Here's how the part is built. I have some questions about the finished solid (model axes, mm). Face numbers are marked on the shaded views. A direction names the side the tool comes from. Coordinates: 2 decimals unless noted, no trailing zeros. Write each loop counter-clockwise with the first axis right and the second up, starting at its lowest first coordinate (ties: lowest second). Pieces come first, ordered by that corner, then holes.
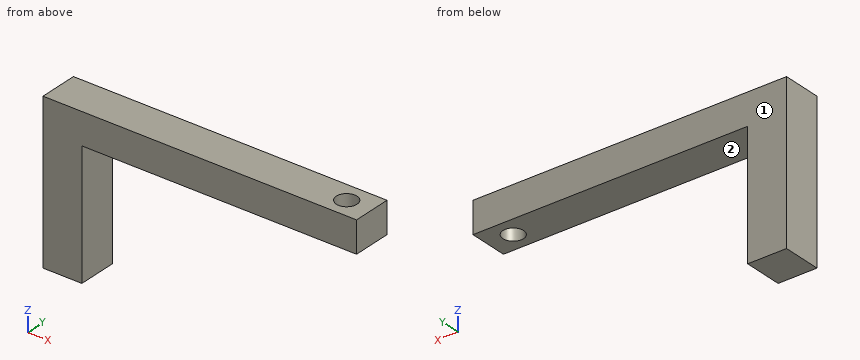
from build123d import *

# Parameters (mm, degrees)
F0_W     = 6.2
F0_H     = 6.2
F1_DEPTH = 20
F2_W     = 50
F2_H     = 6.2
F3_DEPTH = 5
F4_R     = 1.65
F5_DEPTH = 25


with BuildPart() as f1:
    # F0 (on Top) → F1 (new body)
    with BuildSketch(Plane.XY):
        Rectangle(F0_W, F0_H)
    extrude(amount=F1_DEPTH)

    # F2 (on face) → F3 (join)
    with BuildSketch(Plane.XY.offset(20)):
        with Locations((21.9, 0)):
            Rectangle(F2_W, F2_H)
    extrude(amount=F3_DEPTH)

    # F4 (on face) → F5 (cut)
    with BuildSketch(Plane.XY.offset(25)):
        with Locations((42.9, 0)):
            Circle(F4_R)
    extrude(amount=-F5_DEPTH, mode=Mode.SUBTRACT)


solid = f1.part
1. I want a section at B-B (x = 42.9). List the corners of the cut face in (y, z) for me.
2. On a 3-axis mill with a long thin cutter (end or side, diameter ignored), from which of +Z, -Z, +X, -X, +Y, -Y can I reach the whole of each face in a straight line? I mean the marked faces 1 and 2. Say none if no direction works.
3. If I drill on line 1 (Y direction, x = 42.9, z = 22.75); line 2 (X direction, y = -2.75, z = 8.5); line 3 (Z direction, x = 23, y = -0.75), over which ranges is the centre line in solid material (lowest first)?
4. I want a section at A-A (y = 0). List the corners of the cut face in (x, z) for me, then the cut area to 4 significant figures.
5. I want a section at D-D (y = -2.5). List the corners of the cut face in (x, z) for me.
6. I want a section at C-C (z = 20.75). List the corners of the cut face in (x, y) for me, then the cut area to 3 significant figures.
7. For pin 1 Ø1.9 at (y, z) = (0.5, 14.5) entering from +X; pin 2 Ø3 at (x, y) = (23, 1) entering from -Z, each with a flat end and sliding along its axis, tell me the tip position at first contact or that it passes through.
Response values:
1. outline: (-3.1, 20) - (-1.65, 20) - (-1.65, 25) - (-3.1, 25) - close; (1.65, 20) - (3.1, 20) - (3.1, 25) - (1.65, 25) - close
2. face 1: +Z, -Z, +X, -X, +Y
2. face 2: -Z, +X, +Y, -Y
3. line 1: y = -3.1 to -1.65, 1.65 to 3.1
3. line 2: x = -3.1 to 3.1
3. line 3: z = 20 to 25
4. outline: (-3.1, 0) - (3.1, 0) - (3.1, 20) - (41.25, 20) - (41.25, 25) - (-3.1, 25) - close; (44.55, 20) - (46.9, 20) - (46.9, 25) - (44.55, 25) - close
4. area: 357.5 mm2
5. outline: (-3.1, 0) - (3.1, 0) - (3.1, 20) - (46.9, 20) - (46.9, 25) - (-3.1, 25) - close
6. outline: (-3.1, -3.1) - (46.9, -3.1) - (46.9, 3.1) - (-3.1, 3.1) - close; hole circle Ø3.3 at (42.9, 0)
6. area: 301 mm2
7. pin 1: stops at x = 3.1
7. pin 2: stops at z = 20
